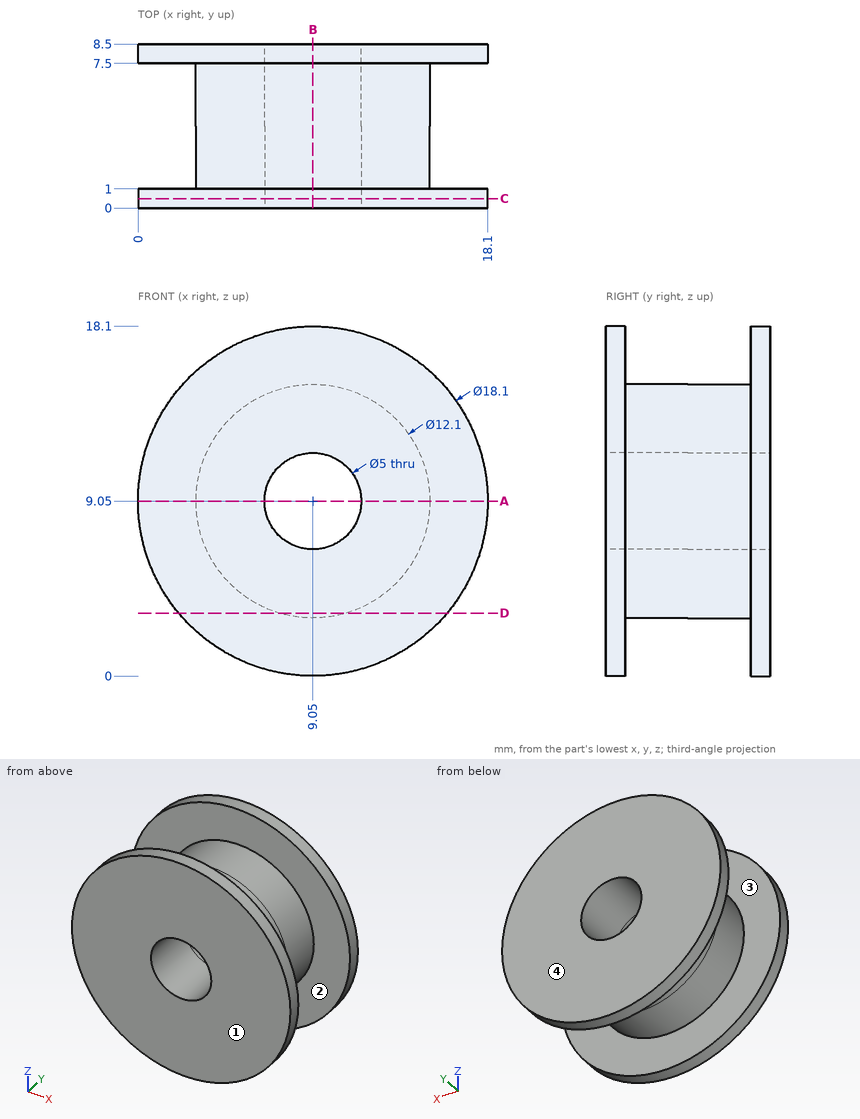
Study the drawing (mm; zero at the part's minimum x, y, z) and answer. Coordinates: 2 decimals unless noted, no trailing zeros. Write each loop counter-clockwise with the first axis right and the second up, starting at its lowest first coordinate (ties: lowest second). Pieces come first, ordered by that corner, then holes. Notation, with made-up numbers: (68.5, 29.25) - (92.5, 29.25) arc R18 ccw to (92.5, 42.25) - close; hole circle Ø9 at (79.25, -23.5). An arc over 180 degrees is marked (long way). Put each result on its own line as item: value.
1. The part is cut by section A-A on z = 9.05. Give the vertices of the cut face in (x, y), plus the area to 4 significant figures.
Answer sheet:
outline: (0, 0) - (6.55, 0) - (6.55, 8.5) - (0, 8.5) - (0, 7.5) - (3, 7.5) - (3, 1) - (0, 1) - close; (11.55, 0) - (18.1, 0) - (18.1, 1) - (15.1, 1) - (15.1, 7.5) - (18.1, 7.5) - (18.1, 8.5) - (11.55, 8.5) - close
area: 72.35 mm^2
2. Find the intervals of material crossed by line 1 along Z through (x, y) = (9.05, 1.45); line 2 along Y through (x, z) = (2, 8.75), in increasing order. Write a range as from..to.
Answer sheet:
line 1: z = 3..6.55, 11.55..15.1
line 2: y = 0..1, 7.5..8.5
3. The part is cut by section D-D on z = 3.25. Give the vertices of the cut face in (x, y).
Answer sheet:
outline: (2.1, 0) - (16, 0) - (16, 1) - (10.77, 1) - (10.77, 7.5) - (16, 7.5) - (16, 8.5) - (2.1, 8.5) - (2.1, 7.5) - (7.33, 7.5) - (7.33, 1) - (2.1, 1) - close
4. The part is cut by section C-C on y = 0.5. Give the vertices of the cut face in (x, z).
Answer sheet:
outline: circle Ø18.1 at (9.05, 9.05); hole circle Ø5 at (9.05, 9.05)
5. Determine the mould class of the marked faces 1, 2, 3 and 4 for opening direction Y: pulls with the +Y half, pulls with the -Y half, needs draft (parallel to the pull), parting line crosses it, or undercut.
Answer sheet:
face 1: pulls with the -Y half
face 2: undercut
face 3: undercut
face 4: pulls with the +Y half
6. The part is cut by section B-B on x = 9.05. Give the vertices of the cut face in (y, z), plus the area to 4 significant figures.
Answer sheet:
outline: (0, 0) - (1, 0) - (1, 3) - (7.5, 3) - (7.5, 0) - (8.5, 0) - (8.5, 6.55) - (0, 6.55) - close; (0, 11.55) - (8.5, 11.55) - (8.5, 18.1) - (7.5, 18.1) - (7.5, 15.1) - (1, 15.1) - (1, 18.1) - (0, 18.1) - close
area: 72.35 mm^2
7. Flat-ended cylindrical pins translate along their axes: pin 1 Ø5 at (x, y) = (4.5, 4.5) entering from -Z; pin 2 Ø8 at (x, z) = (9.05, 9.05) entering from +Y; pin 3 Ø2 at (x, y) = (12.5, 1.5) entering from -Z; pin 4 Ø1 at (x, y) = (14.5, 2.5) entering from +Z. Find the tip coordinate at first contact, or state that the pin passes through.
Answer sheet:
pin 1: stops at z = 3.36
pin 2: stops at y = 8.5
pin 3: stops at z = 0.38
pin 4: stops at z = 12.53
